from build123d import *

# Parameters (mm, degrees)
SKETCH_1_R           = 2.5
EXTRUDE_1_DEPTH      = 5
SKETCH_2_R           = 7.5
EXTRUDE_2_DEPTH      = 5
SKETCH_3_R           = 4.25
EXTRUDE_3_DEPTH      = 5.1
SKETCH_4_R           = 2.25
CUT_EXTRUDE_1_DEPTH  = 36.1
HOLE_WIZARD_M1_8_1_D = 2.1


with BuildPart() as part:
    # 스케치1 → 보스-돌출1 (new body)
    with BuildSketch(Plane.XY):
        with BuildLine():
            Line((0, 10.5), (30, 7.5))
            ThreePointArc((30, 7.5), (37.5, 0), (30, -7.5))
            Line((30, -7.5), (0, -10.5))
            ThreePointArc((0, -10.5), (-10.5, 0), (0, 10.5))
        make_face()
        Circle(SKETCH_1_R, mode=Mode.SUBTRACT)
    extrude(amount=EXTRUDE_1_DEPTH)

    # 스케치2 → 보스-돌출2 (add)
    with BuildSketch(Plane.XY.offset(5)):
        with Locations(Location((30, 0, 0), (0, 0, 90))):
            Circle(SKETCH_2_R)
    extrude(amount=EXTRUDE_2_DEPTH)

    # 스케치3 → 보스-돌출3 (add)
    with BuildSketch(Plane.XY.offset(10)):
        with Locations((30, 0)):
            Circle(SKETCH_3_R)
    extrude(amount=EXTRUDE_3_DEPTH)

    # 스케치4 → 컷-돌출1 (cut)
    with BuildSketch(Plane.XY.offset(15.1)):
        with Locations((30, 0)):
            Circle(SKETCH_4_R)
    extrude(amount=-CUT_EXTRUDE_1_DEPTH, mode=Mode.SUBTRACT)

    # M1.8 여유 구멍1 (through all)
    with Locations(Plane(origin=(0, 0, 0), x_dir=(-1, 0, 0), z_dir=(0, 0, -1))):
        with Locations((2.897458491, -7.322595938), (-7.322595938, -2.897458491), (7.322595938, 2.897458491), (-2.897458491, 7.322595938)):
            Hole(HOLE_WIZARD_M1_8_1_D / 2)


solid = part.part
Part model, mm, in its own coordinate system. A direction names the side the tool comes from. Coordinates: 2 decimals unless noted, no trailing zeros. Loops run counter-clockwise (first coordinate to the right, second up) from the corner with the lowest first, then second, coordinate; pieces in that order, holes last. Notation, with made-up numbers: (48, 45) -> (95, 45) arc R25 cw to (95, 81) -> close; hole circle Ø11 at (54, 8). An arc over 180 degrees is marked (long way). Use a Markdown table: item, result. Add a question column.
Item 1: Flat gauge pins, fed straight in: P1, Ø1.3, axis at x = -2.9, y = -7.32, coming from the -Z side; P2, Ø3, axis at y = 2, z = 4.5, coming from the +X side; P3, Ø3.5, axis at x = -7.32, y = 2.9, coming from the +Z side; P4, Ø1, axis at y = 4.5, z = 8, coming from the +X side. Where does each tip first touch, or does it go through?
Item 2: Band-saw the part on C-C on x = 20. Write the cut outline in (y, z), plus the area to 3 significant figures.
Item 3: Band-saw the part on A-A on y = 0. Write the cut outline in (x, z), plus the area to 3 significant figures.
Item 4: Band-saw the part on B-B on z = 1.5. Write the cut outline in (x, y), plus the area to 3 significant figures.
Item 5: Probe probe 1 along Y at (x, z) = (30, 3.25); probe 2 along X at (y, z) = (2, 1.25); probe 3 along X at (y, z) = (-1.5, 13.25). List the from-to ranges inside material, lowest first.
Item 6: Band-saw the part on D-D on z = 8. Write the cut outline in (x, y).
Item 7: Which spindle directions (+Z, -Z, +X, -X, +Y, -Y) get a long thin tool onto all of the face, cutting with end or side? Do faces 4 (the cylindrical face through (-6.35, 2.5, 2.54)), 5 (the flat face through (33.2, 3.2, 10)). Say none if no direction does.
Item 8: Pull direction Y, two halves, no side cores. Call faces 1 (the flat face through (15, -9, 2)), 2 (the cylindrical face through (-10.5, -0.2, 2.5)), 3 (the cylindrical face through (-0.54, -2.44, 2.46)): +Y half, -Y half, draft (parallel to the pull), parting line (faces both ways), or undercut.
Geometry says:
| question | item | result |
|---|---|---|
| 1 | P1 | through |
| 1 | P2 | x = 37.48 |
| 1 | P3 | z = 5 |
| 1 | P4 | x = 36.34 |
| 2 | outline | (-8.5, 0) -> (8.5, 0) -> (8.5, 5) -> (-8.5, 5) -> close |
| 2 | area | 85.0 mm² |
| 3 | outline | (-10.5, 0) -> (-2.5, 0) -> (-2.5, 5) -> (-10.5, 5) -> close; (2.5, 0) -> (27.75, 0) -> (27.75, 15.1) -> (25.75, 15.1) -> (25.75, 10) -> (22.5, 10) -> (22.5, 5) -> (2.5, 5) -> close; (32.25, 0) -> (37.5, 0) -> (37.5, 10) -> (34.25, 10) -> (34.25, 15.1) -> (32.25, 15.1) -> close |
| 3 | area | 265 mm² |
| 4 | outline | (0, -10.5) -> (30, -7.5) arc R7.5 ccw to (30, 7.5) -> (0, 10.5) arc R10.5 ccw to start; hole circle Ø2.1 at (-7.32, 2.9); hole circle Ø2.1 at (-2.9, -7.32); hole circle Ø5 at (0, 0); hole circle Ø2.1 at (2.9, 7.32); hole circle Ø2.1 at (7.32, -2.9); hole circle Ø4.5 at (30, 0) |
| 4 | area | 752 mm² |
| 5 | probe 1 | -7.5 to -2.25, 2.25 to 7.5 |
| 5 | probe 2 | -10.31 to -7.87, -6.78 to -1.5, 1.5 to 28.97, 31.03 to 37.23 |
| 5 | probe 3 | 26.02 to 28.32, 31.68 to 33.98 |
| 6 | outline | circle Ø15 at (30, 0); hole circle Ø4.5 at (30, 0) |
| 7 | face 4 | +Z, -Z |
| 7 | face 5 | +Z |
| 8 | face 1 | -Y half |
| 8 | face 2 | parting line |
| 8 | face 3 | undercut |
